```python
from build123d import *

# Parameters (mm, degrees)
SKETCH_1_R          = 19
SKETCH_1_R_2        = 16
EXTRUDE_1_DEPTH     = 63.5
SKETCH_2_R          = 12.3
SKETCH_2_R_2        = 10
EXTRUDE_2_DEPTH     = 38
SKETCH_3_R          = 16
CUT_EXTRUDE_1_DEPTH = 64.5000001
CUT_EXTRUDE_2_REACH = 59
SKETCH_7_R          = 10


with BuildPart() as part:
    # 草图1 → 凸台-拉伸1 (new body)
    with BuildSketch(Plane(origin=(0, 0, 0), x_dir=(1, 0, 0), z_dir=(0, 1, 0))):
        Circle(SKETCH_1_R)
        Circle(SKETCH_1_R_2, mode=Mode.SUBTRACT)
    extrude(amount=EXTRUDE_1_DEPTH)

    # 草图2 → 凸台-拉伸2 (add)
    with BuildSketch(Plane.XY):
        with Locations((0, 31.75)):
            Circle(SKETCH_2_R)
        with Locations((0, 31.75)):
            Circle(SKETCH_2_R_2, mode=Mode.SUBTRACT)
    extrude(amount=EXTRUDE_2_DEPTH)

    # 草图3 → 切除-拉伸1 (cut, through all)
    with BuildSketch(Plane.XZ):
        Circle(SKETCH_3_R)
    extrude(amount=-CUT_EXTRUDE_1_DEPTH, mode=Mode.SUBTRACT)

    # 草图7 → 切除-拉伸2 (cut, up to next)
    with BuildSketch(Plane.XY.offset(38), mode=Mode.PRIVATE) as cut_extrude_2_sk1:
        with Locations((0, 31.75)):
            Circle(SKETCH_7_R)
    cut_extrude_2_tool1 = extrude(cut_extrude_2_sk1.sketch, amount=-CUT_EXTRUDE_2_REACH, mode=Mode.PRIVATE) & part.part
    add(cut_extrude_2_tool1.solids().sort_by_distance((0, 31.75, 38))[0], mode=Mode.SUBTRACT)


solid = part.part
```
Source: CAD feature listing. Evaluate the final solid. Frame: model axes, mm. A direction names the side the tool comes from. Coordinates: 2 decimals unless noted, no trailing zeros. Loops run counter-clockwise (first coordinate to the right, second up) from the corner with the lowest first, then second, coordinate; pieces in that order, holes last. Notation, with made-up numbers: M 7,55.25 L 28,55.25 A24 cw 28,77.25 Z; hole C 52,-11 d4. An arc over 180 degrees is marked long. Use a Markdown table: item, result. Add a question column.
Q1. Section query D-D, the plane y = 46. Return loops of the section in (x, z), and give its area (3 significant figures).
Q2. Section query B-B, the plane x = 0. Return loops of the section in (y, z), and give its area (3 significant figures).
Q3. Access query for faces 1 (the flat face through (-10, 0, 13)), 2 (the cylindrical face through (11.362, 27.039, 26.076)). Directions: +Z, -Z, +X, -X, +Y, -Y. A direction counts if a zero-diameter tool reaches every point of the face in a straight line with its end or side. Return the directions, or none.
Q4. Material intervals for L1, parallel to X at y = 33.5, z = 0; L2, parallel to Y at x = 0, z = 27.25; L3, parallel to Z at x = 12, y = 50, sorted ascending.
Q5. Section query C-C, the plane x = 14. Return loops of the section in (y, z), and give its area (3 significant figures).
Q6. First-contact query: pin 1 (1.5 mm diameter, centred on y = 51.5, z = -7, fed in from -X); pin 2 (1.5 mm diameter, centred on y = 55.5, z = -10, fed in from +X); pin 3 (4 mm diameter, centred on x = -6, z = 32, fed in from +Y). Flat tips, straight axial feed; report the tip coordinate or a pass-through.
Q7. Section query A-A, the plane z = 0. Return loops of the section in (x, y).
Result:
| question | item | result |
|---|---|---|
| 1 | outline | C 0,0 d38; hole C 0,0 d32 |
| 1 | area | 330 mm2 |
| 2 | outline | M 0,-19 L 63.5,-19 L 63.5,-16 L 0,-16 Z; M 0,16 L 21.75,16 L 21.75,38 L 19.45,38 L 19.45,19 L 0,19 Z; M 41.75,16 L 63.5,16 L 63.5,19 L 44.05,19 L 44.05,38 L 41.75,38 Z |
| 2 | area | 408 mm2 |
| 3 | face 1 | +Z, -Z, +X, -X, -Y |
| 3 | face 2 | +Z |
| 4 | L1 | x = -19 to -16, 16 to 19 |
| 4 | L2 | y = 19.45 to 21.75, 41.75 to 44.05 |
| 4 | L3 | z = -14.73 to -10.58, 10.58 to 14.73 |
| 5 | outline | M 0,-12.85 L 63.5,-12.85 L 63.5,-7.75 L 0,-7.75 Z; M 0,7.75 L 63.5,7.75 L 63.5,12.85 L 0,12.85 Z |
| 5 | area | 648 mm2 |
| 6 | pin 1 | stops at x = -17.94 |
| 6 | pin 2 | stops at x = 16.6 |
| 6 | pin 3 | stops at y = 43.38 |
| 7 | outline | M -19,0 L -16,0 L -16,63.5 L -19,63.5 Z; M 16,0 L 19,0 L 19,63.5 L 16,63.5 Z |
